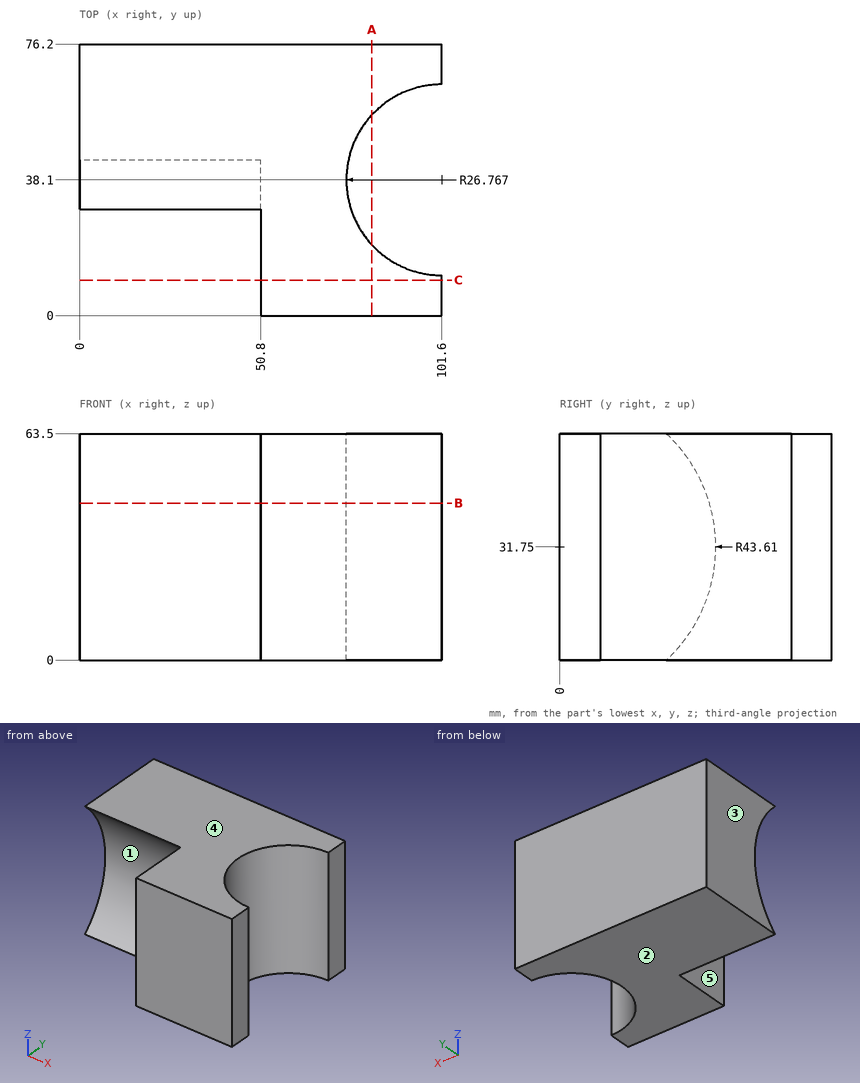
Geometry: see drawing. Coordinates: mm, zero at the bounding-box minimum. A direction names the side the tool comes from. Round coordinates to 2 decimals unless told otherwise and drop trailing zeros. Loops run counter-clockwise (first coordinate to the right, second up) from the corner with the lowest first, then second, coordinate; pieces in that order, holes last. Notation, with made-up numbers: M -16.75,24.5 L 38.25,24.5 A34 ccw 38.25,62.5 Z; hole C 45.25,-5.5 d6. An arc over 180 degrees is marked long. Use a Markdown table: item, result. Add a question column.
1. Contact query for flat-ended pins moving along their axis: P1, Ø22, axis at y = 13.5, z = 28.5, coming from the -X side; P2, Ø2, axis at x = 87.5, z = 43, coming from the -Y side; P3, Ø12, axis at y = 27.5, z = 32, coming from the +X side; P4, Ø2, axis at y = 23, z = 8, coming from the +X side (1 decimal). Output: stop coordinate, or through.
2. Section query C-C on y = 10. Return the cut outline in (x, z), then the cut area to 3 significant figures.
3. Reachability of the marked faces 4 and 5 from +Z, -Z, +X, -X, +Y, -Y: full face, straight path, thin tool, end or side. Return the list, or none.
4. Section query B-B on z = 44. Return the cut outline in (x, y).
5. Section query A-A on x = 82. Return the cut outline in (y, z), then the cut area to 3 significant figures.
6. Line query: line 1 (Y direction, x = 91.5, z = 36.5); line 2 (Y direction, x = 84.5, z = 15) (1 decimal); line 3 (Z direction, x = 50, y = 40) (1 decimal). Output: solid intervals per line, ascending.
7. Mould query, pull axis Z, two halves, no side actions, for the marked faces 1, 2 and 3. Classes: pulls with the +Z half, pulls with the -Z half, needs draft (parallel to the pull), parting line crosses it, or undercut.
Reported:
| question | item | result |
|---|---|---|
| 1 | P1 | stops at x = 50.8 |
| 1 | P2 | stops at y = 0 |
| 1 | P3 | stops at x = 80.6 |
| 1 | P4 | stops at x = 80.2 |
| 2 | outline | M 50.8,0 L 101.6,0 L 101.6,63.5 L 50.8,63.5 Z |
| 2 | area | 3,230 mm² |
| 3 | face 4 | +Z, +X, -X, +Y, -Y |
| 3 | face 5 | -X, -Y |
| 4 | outline | M 0,41.85 L 50.8,41.85 L 50.8,0 L 101.6,0 L 101.6,11.33 A26.77 cw 101.6,64.87 L 101.6,76.2 L 0,76.2 Z |
| 5 | outline | M 0,0 L 19.87,0 L 19.87,63.5 L 0,63.5 Z; M 56.33,0 L 76.2,0 L 76.2,63.5 L 56.33,63.5 Z |
| 5 | area | 2,520 mm² |
| 6 | line 1 | y = 0 to 13.31, 62.89 to 76.2 |
| 6 | line 2 | y = 0 to 17.5, 58.7 to 76.2 |
| 6 | line 3 | z = 0 to 14.4, 49.1 to 63.5 |
| 7 | face 1 | undercut |
| 7 | face 2 | pulls with the -Z half |
| 7 | face 3 | needs draft |
